Part model, mm, in its own coordinate system. Face numbers are marked on the shaded views. A direction names the side the tool comes from. Coordinates: 2 decimals unless noted, no trailing zeros. Loops run counter-clockwise (first coordinate to the right, second up) from the corner with the lowest first, then second, coordinate; pieces in that order, holes last. Notation, with made-up numbers: M 74.25,55 L 122.25,55 A23 cw 122.25,85 Z; hole C 87.25,76.5 d1. An arc over 180 degrees is marked long. Use CSV: the item, a comma, the result in double quotes. Start each with the question number.
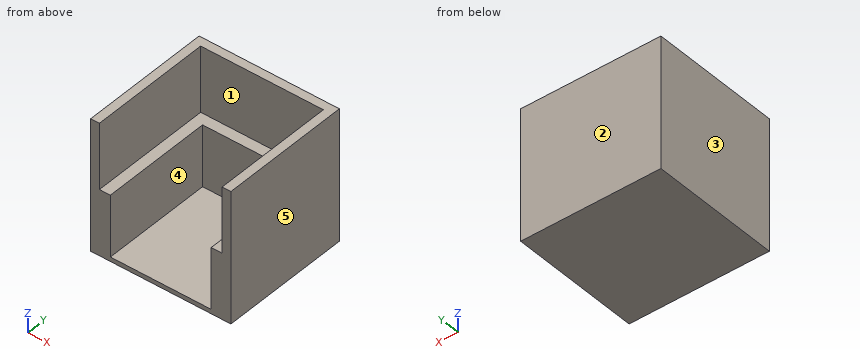
from build123d import *

# Parameters (mm, degrees)
F1_DEPTH = 76.2
F2_W     = 6.35
F2_H     = 71.12
F3_DEPTH = 38.1
F4_W     = 58.42
F4_H     = 71.12
F5_DEPTH = 2.54
F6_W     = 58.42
F6_H     = 6.35
F7_DEPTH = 38.1


with BuildPart() as f1:
    # F0 (on Top) → F1 (new body)
    with BuildSketch(Plane.XY):
        Polygon((-27.812527, 51.794526), (-27.812527, -24.405474), (-22.732527, -24.405474), (-22.732527, 46.714526), (48.387473, 46.714526), (48.387473, -24.405474), (53.467473, -24.405474), (53.467473, 51.794526), align=None)
    extrude(amount=F1_DEPTH)

    # F2 (on Top) → F3 (join)
    with BuildSketch(Plane.XY):
        with Locations((-19.557527, 11.154526)):
            Rectangle(F2_W, F2_H)
        with Locations((45.212473, 11.154526)):
            Rectangle(F2_W, F2_H)
    extrude(amount=F3_DEPTH)

    # F4 (on Top) → F5 (join)
    with BuildSketch(Plane.XY):
        with Locations((12.827473, 11.154526)):
            Rectangle(F4_W, F4_H)
    extrude(amount=F5_DEPTH)

    # F6 (on Top) → F7 (join)
    with BuildSketch(Plane.XY):
        with Locations((12.827473, 43.539526)):
            Rectangle(F6_W, F6_H)
    extrude(amount=F7_DEPTH)


solid = f1.part
1. Two-plate mould, pull along X, no slides. Class the marked faces 1, 2 and 3: pulls with the +X half, pulls with the -X half, needs draft (parallel to the pull), parting line crosses it, or undercut.
2. Wall check: probe 1 along X at (y, z) = (-7, 64); probe 2 along X at (y, z) = (-13.5, 19.5); probe 3 along Z at (x, y) = (11, -0.5). Give the ranges that are in metal, low to high.
3. Tool access for the marked faces 4 and 5: list every direction of +Z, -Z, +X, -X, +Y, -Y with a clear straight run to the whole face (end or side of a thin tool).
4. Slice it at B-B, the plane z = 52.5. List the corners of the cut face in (x, y).
5. Slice it at C-C, the plane x = 36. List the corners of the cut face in (y, z), and give its area (3 significant figures).
6. Pin check, flat tips, straight feed: pin 1 (11.5 mm diameter, centred on x = 10.5, z = 63.5, fed in from -Y); pin 2 (5 mm diameter, centred on x = -18.5, y = 32, fed in from +Z); pin 3 (21.5 mm diameter, centred on x = 20, y = 26, fed in from +Z). Stop position of each tip, or through.
7. Slice it at A-A, the plane y = 6.5. List the corners of the cut face in (x, z), and give its area (3 significant figures).
Found:
1,face 1,"undercut"
1,face 2,"needs draft"
1,face 3,"pulls with the -X half"
2,probe 1,"-27.81 to -22.73, 48.39 to 53.47"
2,probe 2,"-27.81 to -16.38, 42.04 to 53.47"
2,probe 3,"0 to 2.54"
3,face 4,"+Z, -Y"
3,face 5,"+Z, -Z, +X, +Y, -Y"
4,outline,"M -27.81,-24.41 L -22.73,-24.41 L -22.73,46.71 L 48.39,46.71 L 48.39,-24.41 L 53.47,-24.41 L 53.47,51.79 L -27.81,51.79 Z"
5,outline,"M -24.41,0 L 51.79,0 L 51.79,76.2 L 46.71,76.2 L 46.71,38.1 L 40.36,38.1 L 40.36,2.54 L -24.41,2.54 Z"
5,area,"794 mm^2"
6,pin 1,"y = 46.71"
6,pin 2,"z = 38.1"
6,pin 3,"z = 2.54"
7,outline,"M -27.81,0 L 53.47,0 L 53.47,76.2 L 48.39,76.2 L 48.39,38.1 L 42.04,38.1 L 42.04,2.54 L -16.38,2.54 L -16.38,38.1 L -22.73,38.1 L -22.73,76.2 L -27.81,76.2 Z"
7,area,"1,410 mm^2"
